from build123d import *

# Parameters (mm, degrees)
BOSS_EXTRUDE1_DEPTH                          = 20
CSK_FOR_M3_COUNTERSUNK_FLAT_HEAD_SCR_2_COUNT = 2
CSK_FOR_M3_COUNTERSUNK_FLAT_HEAD_SCR_2_PITCH = 35
CSK_FOR_M3_COUNTERSUNK_FLAT_HEAD_SCR_3_COUNT = 2
CSK_FOR_M3_COUNTERSUNK_FLAT_HEAD_SCR_3_PITCH = 10
CSK_FOR_M3_COUNTERSUNK_FLAT_HEAD_SCR_4_COUNT = 2
CSK_FOR_M3_COUNTERSUNK_FLAT_HEAD_SCR_4_PITCH = 36.400549446


with BuildPart() as part:
    # Sketch1 → Boss-Extrude1 (new body)
    with BuildSketch(Plane(origin=(0, 0, 0), x_dir=(1, 0, 0), z_dir=(0, 1, 0))):
        with BuildLine():
            Line((-7.62, 0), (-22.5, 0))
            Line((-22.5, 0), (-22.5, 1.5))
            Line((-22.5, 1.5), (-8.99579902, 1.5))
            ThreePointArc((-8.99579902, 1.5), (0, 9.12), (8.99579902, 1.5))
            Line((8.99579902, 1.5), (22.5, 1.5))
            Line((22.5, 1.5), (22.5, 0))
            Line((22.5, 0), (7.62, 0))
            ThreePointArc((7.62, 0), (0, 7.62), (-7.62, 0))
        make_face()
    extrude(amount=BOSS_EXTRUDE1_DEPTH)

    # Sketch3 → CSK for M3 Countersunk Flat Head Screw1 (revolve, cut)
    with BuildSketch(Plane(origin=(17.5, 5, -1.5), x_dir=(0, 1, 0), z_dir=(1, 0, 0))):
        Polygon((0, 0), (0, 1.5), (1.7, 1.5), (1.7, 1.45), (3.15, 0), align=None)
    csk_for_m3_countersunk_flat_head_screw1 = revolve(axis=Axis((17.5, 5, -7.85), (0, 0, 1)), mode=Mode.SUBTRACT)

    # CSK for M3 Countersunk Flat Head Scr 2: CSK for M3 Countersunk Flat Head Screw1 ×2
    with Locations(*[(-i * CSK_FOR_M3_COUNTERSUNK_FLAT_HEAD_SCR_2_PITCH, 0, 0) for i in range(1, CSK_FOR_M3_COUNTERSUNK_FLAT_HEAD_SCR_2_COUNT)]):
        add(csk_for_m3_countersunk_flat_head_screw1, mode=Mode.SUBTRACT)

    # CSK for M3 Countersunk Flat Head Scr 3: CSK for M3 Countersunk Flat Head Screw1 ×2
    with Locations(*[(0, i * CSK_FOR_M3_COUNTERSUNK_FLAT_HEAD_SCR_3_PITCH, 0) for i in range(1, CSK_FOR_M3_COUNTERSUNK_FLAT_HEAD_SCR_3_COUNT)]):
        add(csk_for_m3_countersunk_flat_head_screw1, mode=Mode.SUBTRACT)

    # CSK for M3 Countersunk Flat Head Scr 4: CSK for M3 Countersunk Flat Head Screw1 ×2
    with Locations(*[Vector(-0.9615239476408232, 0.27472112789737807, 0) * (i * CSK_FOR_M3_COUNTERSUNK_FLAT_HEAD_SCR_4_PITCH) for i in range(1, CSK_FOR_M3_COUNTERSUNK_FLAT_HEAD_SCR_4_COUNT)]):
        add(csk_for_m3_countersunk_flat_head_screw1, mode=Mode.SUBTRACT)


solid = part.part
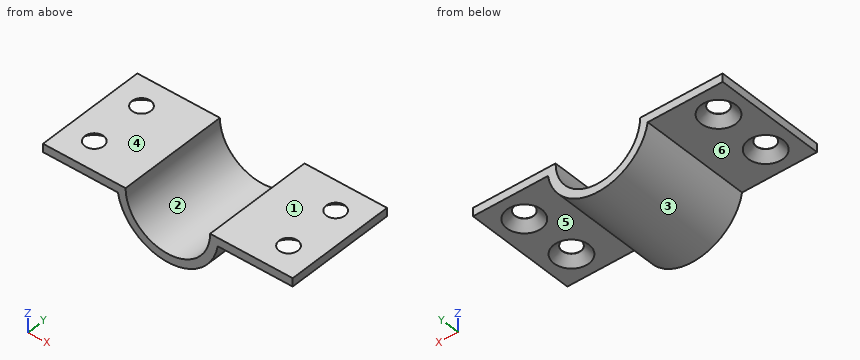
Verification items for the finished model (mm, model axes). Face numbers are marked on the shaded views. A direction names the side the tool comes from. Give positions to 0.01 mm unless a question says otherwise; leave off trailing zeros. Loops run counter-clockwise (first coordinate to the right, second up) from the corner with the lowest first, then second, coordinate; pieces in that order, holes last.
1. Cross-section at B-B on y = 15. Record the cut outline in (x, z), and give its area (3 significant figures).
Derived:
outline: (-22.5, -1.5) - (-20.65, -1.5) - (-19.2, -0.05) - (-19.2, 0) - (-22.5, 0) - close; (-15.8, -0.05) - (-14.35, -1.5) - (-9, -1.5) arc R9.12 ccw to (9, -1.5) - (14.35, -1.5) - (15.8, -0.05) - (15.8, 0) - (7.62, 0) arc R7.62 cw to (-7.62, 0) - (-15.8, 0) - close; (19.2, -0.05) - (20.65, -1.5) - (22.5, -1.5) - (22.5, 0) - (19.2, 0) - close
area: 65.3 mm2
2. Material ranges on probe 1 along Z at (x, y) = (-15.5, 10.25); probe 2 along X at (y, z) = (10.5, -5); probe 3 along X at (y, z) = (5.5, -6), recorded low to high.
Derived:
probe 1: z = -1.5 to 0
probe 2: x = -7.63 to -5.75, 5.75 to 7.63
probe 3: x = -6.87 to -4.7, 4.7 to 6.87
3. Cross-section at A-A on z = -2.5. Record the cut outline in (x, y).
Derived:
outline: (-8.77, 0) - (-7.2, 0) - (-7.2, 20) - (-8.77, 20) - close; (7.2, 0) - (8.77, 0) - (8.77, 20) - (7.2, 20) - close
4. Release check for a two-part mould opening along X. For the marked faces 1, 2 and 3 record: +X half, -X half, draft (parallel to the pull), parting line (faces both ways), or undercut.
Derived:
face 1: draft
face 2: undercut
face 3: parting line
5. Cross-section at C-C on y = 9.5. Record the cut outline in (x, z), and give its area (3 significant figures).
Derived:
outline: (-22.5, -1.5) - (-9, -1.5) arc R9.12 ccw to (9, -1.5) - (22.5, -1.5) - (22.5, 0) - (7.62, 0) arc R7.62 cw to (-7.62, 0) - (-22.5, 0) - close
area: 79.7 mm2
6. Tool access check on the marked faces 4, 5 and 6. Record the directions out of +Z, -Z, +X, -X, +Y, -Y that give a thin tool (end or side, any length) a straight path to the whole face; none if there is none.
Derived:
face 4: +Z, +X, -X, +Y, -Y
face 5: -Z, +X, +Y, -Y
face 6: -Z, -X, +Y, -Y
7. Cross-section at D-D on x = -10.5. Record the cut outline in (y, z).
Derived:
outline: (0, -1.5) - (20, -1.5) - (20, 0) - (0, 0) - close
8. Go/stop test with flat-tipped pins: P1, Ø5.5, axis at x = -17.5, y = 15, coming from the -Z side; P2, Ø2, axis at x = 17.5, y = 5, coming from the +Z side; P3, Ø3, axis at x = -12, y = 12, coming from the -Z side; P4, Ø1, axis at y = 10.5, z = -3, coming from the -X side. Record where each tip stops, or that it passes through.
Derived:
P1: stops at z = -1.1
P2: passes through
P3: stops at z = -1.5
P4: stops at x = -8.77
